Read the model definition and answer for the solid it produces. Units are mm, in the model's axes. Face numbers are marked on the shaded views. A direction names the side the tool comes from. Round coordinates to 2 decimals unless told otherwise and drop trailing zeros. Write each loop counter-clockwise with the first axis right and the second up, starting at its lowest first coordinate (ties: lowest second). Pieces come first, ordered by that corner, then holes. Notation, with made-up numbers: (59.5, -9) - (112.5, -9) arc R18 ccw to (112.5, -3) - close; hole circle Ø11 at (83.5, 14). An arc over 180 degrees is marked (long way). Use one line per item in the form item = value. Start each with the question number.
1) The part is cut by section B-B, the plane x = -14. Give the vertices of the cut face in (y, z).
2) For the marked faces 4, 5, 6, 7 and 8, determine the directions among +Z, -Z, +X, -X, +Y, -Y from which every point of the face is accessible in a straight line to the end or side of a thin tool.
3) The part is cut by section A-A, the plane y = 0. Give the vertices of the cut face in (x, z).
4) Each of these flat-tipped pins is pushed along its axis until it touches: pin 1 (1.9 mm diameter, centred on x = -14, y = 0, fed in from +Z); pin 2 (6 mm diameter, centred on y = -5.5, z = -6, fed in from +X); pin 3 (0.8 mm diameter, centred on y = -7, z = -5.5, fed in from +X); pin 4 (2 mm diameter, centred on y = -4.5, z = -0.5, fed in from -X). Where does it stop, or does it pass through?
5) The part is cut by section C-C, the plane x = -16. Give the vertices of the cut face in (y, z).
6) Consider line 1 along Z through (x, y) = (-8.5, 5.75); line 2 along Y through (x, z) = (-14, 4.65); line 3 along X through (y, z) = (4, 3). Determine where each line is inside the solid, lowest interval first. Write a range as from..to.
7) The part is cut by section D-D, the plane z = 0. Give the vertices of the cut face in (x, y), plus the area to 3 significant figures.
8) For a pull along Y with two mould halves and no side action, classify the marked faces 1, 2 and 3 as released by +Y, released by -Y, zero draft, split by the parting line, or undercut.
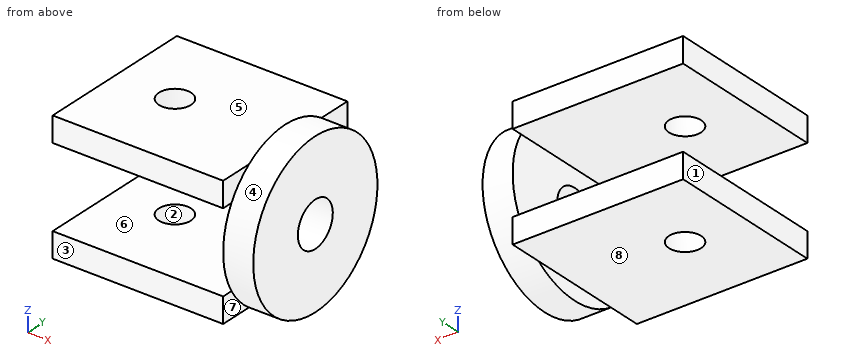
from build123d import *

# Parameters (mm, degrees)
BASE_SKETCH_W        = 3
BASE_SKETCH_H        = 8
CHEEK_BLOCK_SKETCH_W = 17
CHEEK_BLOCK_SKETCH_H = 16
CHEEK_BLOCK_DEPTH    = 6.5
GAP_SKETCH_W         = 18
GAP_SKETCH_H         = 18
GAP_DEPTH            = 4
PIN_HOLE_SKETCH_R    = 1.6
PIN_HOLE_DEPTH       = 8.5
SCREW_HOLE_SKETCH_W  = 4
SCREW_HOLE_SKETCH_H  = 2.25


with BuildPart() as part:
    # Base Sketch → Base (revolve)
    with BuildSketch(Plane.XY, mode=Mode.PRIVATE) as base_sk:
        with Locations((-1.5, 4)):
            Rectangle(BASE_SKETCH_W, BASE_SKETCH_H)
    revolve(base_sk.sketch.rotate(Axis((-3000, 0, 0), (1, 0, 0)), 90), axis=Axis((-3000, 0, 0), (1, 0, 0)))

    # Cheek Block Sketch → Cheek Block (add, symmetric)
    with BuildSketch(Plane.XY):
        with Locations((-11.5, 0)):
            Rectangle(CHEEK_BLOCK_SKETCH_W, CHEEK_BLOCK_SKETCH_H)
    extrude(amount=CHEEK_BLOCK_DEPTH, both=True)

    # Gap Sketch → Gap (cut, symmetric)
    with BuildSketch(Plane.XY):
        with Locations((-12, 0)):
            Rectangle(GAP_SKETCH_W, GAP_SKETCH_H)
    extrude(amount=GAP_DEPTH, both=True, mode=Mode.SUBTRACT)

    # Pin Hole Sketch → Pin Hole (cut, symmetric)
    with BuildSketch(Plane.XY):
        with Locations((-14, 0)):
            Circle(PIN_HOLE_SKETCH_R)
    extrude(amount=PIN_HOLE_DEPTH, both=True, mode=Mode.SUBTRACT)

    # Screw Hole Sketch → Screw Hole (revolve, cut)
    with BuildSketch(Plane.XY, mode=Mode.PRIVATE) as screw_hole_sk:
        with Locations((-1.5, 1.125)):
            Rectangle(SCREW_HOLE_SKETCH_W, SCREW_HOLE_SKETCH_H)
    revolve(screw_hole_sk.sketch.rotate(Axis((-3000, 0, 0), (1, 0, 0)), 90), axis=Axis((-3000, 0, 0), (1, 0, 0)), mode=Mode.SUBTRACT)


solid = part.part
Geometry results:
q1.outline = (-8, -6.5) - (-1.6, -6.5) - (-1.6, -4) - (-8, -4) - close; (-8, 4) - (-1.6, 4) - (-1.6, 6.5) - (-8, 6.5) - close; (1.6, -6.5) - (8, -6.5) - (8, -4) - (1.6, -4) - close; (1.6, 4) - (8, 4) - (8, 6.5) - (1.6, 6.5) - close
q2.face_4 = +X
q2.face_5 = +Z, -X, +Y, -Y
q2.face_6 = -X, +Y, -Y
q2.face_7 = -Z, +X, -Y
q2.face_8 = -Z, -X, +Y, -Y
q3.outline = (-20, -6.5) - (-15.6, -6.5) - (-15.6, -4) - (-20, -4) - close; (-20, 4) - (-15.6, 4) - (-15.6, 6.5) - (-20, 6.5) - close; (-12.4, -6.5) - (-3, -6.5) - (-3, -8) - (0, -8) - (0, -2.25) - (-3, -2.25) - (-3, -4) - (-12.4, -4) - close; (-12.4, 4) - (-3, 4) - (-3, 2.25) - (0, 2.25) - (0, 8) - (-3, 8) - (-3, 6.5) - (-12.4, 6.5) - close
q4.pin_1 = through
q4.pin_2 = 0
q4.pin_3 = -3
q4.pin_4 = -3
q5.outline = (-8, -6.5) - (8, -6.5) - (8, -4) - (-8, -4) - close; (-8, 4) - (8, 4) - (8, 6.5) - (-8, 6.5) - close
q6.line_1 = -6.5..-4, 4..6.5
q6.line_2 = -8..-1.6, 1.6..8
q6.line_3 = -3..0
q7.outline = (-3, -8) - (0, -8) - (0, -2.25) - (-3, -2.25) - close; (-3, 2.25) - (0, 2.25) - (0, 8) - (-3, 8) - close
q7.area = 34.5 mm2
q8.face_1 = zero draft
q8.face_2 = undercut
q8.face_3 = released by -Y
